The model under review builds one solid part; all positions refer to its coordinate system, in mm. A direction names the side the tool comes from. Coordinates: 2 decimals unless noted, no trailing zeros. Loops run counter-clockwise (first coordinate to the right, second up) from the corner with the lowest first, then second, coordinate; pieces in that order, holes last. Notation, with made-up numbers: (25, 61) - (74, 61) arc R26 ccw to (74, 87) - close; hole circle Ø6 at (40.5, -9). An arc over 180 degrees is marked (long way). Answer in a Markdown table with one row per item. Add a question column.
(1) Mouldability with a two-part tool opening along Z and no side actions: class faces 1 (the flat face through (-158.2, 4, -23.4)), 2 (the flat face through (-1, 6, 23)), 3 (the flat face through (-1, 6, 25)) as +Z half, -Z half, draft (parallel to the pull), parting line (faces both ways), or undercut.
(2) Machinability: for faces 4 (the flat face through (158.2, 4, -23.4)), 5 (the flat face through (161.2, 1.6, 17.4)), 6 (the flat face through (-158.2, 4, 23.3)), 7 (the flat face through (-2, 2, 0)), which of the approach directions +Z, -Z, +X, -X, +Y, -Y give a long, thin tool a straight path to every point of the face, cutting with its end or side? Answer none if there is none.
(3) For P1, Ø1.6, axis at x = 165, y = 1.5, coming from the -Z side; P2, Ø5, axis at y = 5, z = 21.5, coming from the -X side; P3, Ø3, axis at y = 2.5, z = 18, coming from the +X side, all flat-tipped, find the tip position at first contact; note any pin that passes through.
(4) For line 1 along Z through (x, y) = (-80.5, 4.5); line 2 along Y through (x, z) = (-65.5, -5); line 3 along X through (y, z) = (1.5, 16.5), list the stretches that pass through material, from the lowest coordinate up.
(5) We need section C-C on z = 16. Write out the cut boundary in (x, y).
(6) We need section A-A on y = 4.5. Write out the cut boundary in (x, z), plus the area to 3 significant figures.
(7) We need section B-B on x = -104.5. Write out the cut boundary in (y, z).
(8) We need section D-D on z = -6.5. Write out the cut boundary in (x, y), plus the area to 3 significant figures.
from build123d import *

# Parameters (mm, degrees)
SKETCH1_W                    = 342.4
SKETCH1_H                    = 50
BASE_FLANGE1_DEPTH           = 2
EDGE_FLANGE1_STRIP_W         = 9.4732
EDGE_FLANGE1_STRIP_H         = 2
EDGE_FLANGE1_STRIP_CUT_DEPTH = 342.4
EDGE_FLANGE1_DEPTH           = 342.4
EDGE_FLANGE2_STRIP_W         = 9.4732
EDGE_FLANGE2_STRIP_H         = 2
EDGE_FLANGE2_STRIP_CUT_DEPTH = 342.4
EDGE_FLANGE2_DEPTH           = 342.4
CUT_EXTRUDE2_DEPTH           = 334.488770426
CUT_EXTRUDE3_DEPTH           = 174.200577366
MOVE_START                   = 158.2
MOVE_FACE1_DEPTH             = 3


# Read off the part's stored shape, not the designer's step: Move Face1
# Sheet-metal steps are written as plain solids
with BuildPart() as part:
    # Sketch1 → Base-Flange1 (new body)
    with BuildSketch(Plane(origin=(0, 0, 0), x_dir=(1, 0, 0), z_dir=(0, 1, 0))):
        Rectangle(SKETCH1_W, SKETCH1_H)
    extrude(amount=BASE_FLANGE1_DEPTH)

    # Edge-Flange1 strip (across the edge) → Edge-Flange1 strip cut (cut)
    with BuildSketch(Plane(origin=(-171.2, 2, 25), x_dir=(0, 0, -1), z_dir=(1, 0, 0))):
        with Locations((-2, -1)):
            Rectangle(EDGE_FLANGE1_STRIP_W, EDGE_FLANGE1_STRIP_H)
    extrude(amount=EDGE_FLANGE1_STRIP_CUT_DEPTH, mode=Mode.SUBTRACT)

    # Edge-Flange1 section (across the edge) → Edge-Flange1 (add)
    with BuildSketch(Plane(origin=(-171.2, 2, 25), x_dir=(0, 0, -1), z_dir=(1, 0, 0))):
        with BuildLine():
            Line((0, 0.7366), (0, 8))
            Line((0, 8), (2, 8))
            Line((2, 8), (2, 0.7366))
            ThreePointArc((2, 0.7366), (2.215745145, 0.215745145), (2.7366, 0))
            Line((2.7366, 0), (2.7366, -2))
            ThreePointArc((2.7366, -2), (0.801531583, -1.198468417), (0, 0.7366))
        make_face()
    extrude(amount=EDGE_FLANGE1_DEPTH)

    # Edge-Flange2 strip (across the edge) → Edge-Flange2 strip cut (cut)
    with BuildSketch(Plane(origin=(171.2, 2, -25), x_dir=(0, 0, 1), z_dir=(-1, 0, 0))):
        with Locations((-2, -1)):
            Rectangle(EDGE_FLANGE2_STRIP_W, EDGE_FLANGE2_STRIP_H)
    extrude(amount=EDGE_FLANGE2_STRIP_CUT_DEPTH, mode=Mode.SUBTRACT)

    # Edge-Flange2 section (across the edge) → Edge-Flange2 (add)
    with BuildSketch(Plane(origin=(171.2, 2, -25), x_dir=(0, 0, 1), z_dir=(-1, 0, 0))):
        with BuildLine():
            Line((0, 0.7366), (0, 8))
            Line((0, 8), (2, 8))
            Line((2, 8), (2, 0.7366))
            ThreePointArc((2, 0.7366), (2.215745145, 0.215745145), (2.7366, 0))
            Line((2.7366, 0), (2.7366, -2))
            ThreePointArc((2.7366, -2), (0.801531583, -1.198468417), (0, 0.7366))
        make_face()
    extrude(amount=EDGE_FLANGE2_DEPTH)

    # Sketch18 → Cut-Extrude2 (cut, through all)
    with BuildSketch(Plane(origin=(161.2, 0, 0), x_dir=(0, 0, -1), z_dir=(1, 0, 0))):
        Polygon((-3.3, 6.000000001), (-3.3, 10.000000001), (-37.658134746, 10.000000001), (-37.658134746, -5.535311506), (-3.3, -5.535311506), align=None)
    extrude(amount=CUT_EXTRUDE2_DEPTH, mode=Mode.SUBTRACT)

    # Sketch19 → Cut-Extrude3 (cut, symmetric)
    with BuildSketch(Plane(origin=(0, 2, 0), x_dir=(1, 0, 0), z_dir=(0, 1, 0))):
        Polygon((-249.45231786, 85.285820153), (-158.2, 85.285820153), (-158.2, 19), (-209.845513649, 19), (-209.845513649, -19), (-158.2, -19), (-158.2, -89.848436046), (-249.45231786, -89.848436046), align=None)
    cut_extrude3 = extrude(amount=CUT_EXTRUDE3_DEPTH, both=True, mode=Mode.SUBTRACT)

    # Mirror1: Cut-Extrude3 across plane
    add(cut_extrude3.mirror(Plane(origin=(0, 0, 0), x_dir=(0, 0, 1), z_dir=(1, 0, 0))), mode=Mode.SUBTRACT)

    # Move Face1 outline → Move Face1 (add)
    with BuildSketch(Plane.YZ.offset(MOVE_START)):
        with BuildLine():
            Line((0, 19), (2, 19))
            Line((2, 19), (2, 22.2634))
            ThreePointArc((2, 22.2634), (2.215745145, 22.784254855), (2.7366, 23))
            Line((2.7366, 23), (10.000000001, 23))
            Line((10.000000001, 23), (10, 25))
            Line((10, 25), (2.7366, 25))
            ThreePointArc((2.7366, 25), (0.801531583, 24.198468417), (0, 22.2634))
            Line((0, 22.2634), (0, 19))
        make_face()
    extrude(amount=MOVE_FACE1_DEPTH)


solid = part.part
Outcome:
| question | item | result |
|---|---|---|
| 1 | face 1 | draft |
| 1 | face 2 | undercut |
| 1 | face 3 | +Z half |
| 2 | face 4 | -Z, +X, +Y, -Y |
| 2 | face 5 | +Z, +X, +Y, -Y |
| 2 | face 6 | +Z, -X, +Y, -Y |
| 2 | face 7 | +X, -X, +Y |
| 3 | P1 | z = -19 |
| 3 | P2 | x = -158.2 |
| 3 | P3 | x = 161.2 |
| 4 | line 1 | -25 to -23, 23 to 25 |
| 4 | line 2 | 0 to 2 |
| 4 | line 3 | -171.2 to 161.2 |
| 5 | outline | (-171.2, 0) - (161.2, 0) - (161.2, 2) - (-171.2, 2) - close |
| 6 | outline | (-158.2, -25) - (158.2, -25) - (158.2, -23) - (-158.2, -23) - close; (-158.2, 23) - (161.2, 23) - (161.2, 25) - (-158.2, 25) - close |
| 6 | area | 1,270 mm² |
| 7 | outline | (0, -22.26) arc R2.74 ccw to (2.74, -25) - (10, -25) - (10, -23) - (2.74, -23) arc R0.74 cw to (2, -22.26) - (2, 22.26) arc R0.74 cw to (2.74, 23) - (10, 23) - (10, 25) - (2.74, 25) arc R2.74 ccw to (0, 22.26) - close |
| 8 | outline | (-171.2, 0) - (171.2, 0) - (171.2, 2) - (-171.2, 2) - close |
| 8 | area | 685 mm² |
